The listing builds one solid part. Answer for the finished solid, in the listing's coordinates (mm). A direction names the side the tool comes from. Give positions to 0.01 mm unless a question says otherwise; leave off trailing zeros. Order: outer loops, then holes, each group sorted by start corner. A loop starts at its lowest first (then second) coordinate and runs counter-clockwise, first axis right, second up.
```python
from build123d import *

# Parameters (mm, degrees)
SM_BASE_FLANGE_1_DEPTH = 15
CUT_EXTRUDE_1_DEPTH    = 10
FILLET_1_R             = 5


# Sheet-metal steps are written as plain solids
with BuildPart() as part:
    # Sketch 1 → 基体-法兰1 (new, symmetric)
    with BuildSketch(Plane.XY):
        with BuildLine():
            Line((204, 72), (204, 6))
            ThreePointArc((204, 6), (202.242640687, 1.757359313), (198, 0))
            Line((198, 0), (-198, 0))
            ThreePointArc((-198, 0), (-202.242640687, 1.757359313), (-204, 6))
            Line((-204, 6), (-204, 72))
            Line((-204, 72), (-210, 72))
            Line((-210, 72), (-210, 6))
            ThreePointArc((-210, 6), (-206.485281374, -2.485281374), (-198, -6))
            Line((-198, -6), (198, -6))
            ThreePointArc((198, -6), (206.485281374, -2.485281374), (210, 6))
            Line((210, 6), (210, 72))
            Line((210, 72), (204, 72))
        make_face()
    extrude(amount=SM_BASE_FLANGE_1_DEPTH, both=True)

    # 草图6 → 切除-拉伸1 (cut)
    with BuildSketch(Plane.XZ.offset(6)):
        with BuildLine():
            Line((13.5, 7.5), (124.5, 7.5))
            ThreePointArc((124.5, 7.5), (132, 0), (124.5, -7.5))
            Line((124.5, -7.5), (13.5, -7.5))
            ThreePointArc((13.5, -7.5), (6, 0), (13.5, 7.5))
        make_face()
        with BuildLine():
            Line((-13.5, 7.5), (-124.5, 7.5))
            ThreePointArc((-124.5, 7.5), (-132, 0), (-124.5, -7.5))
            Line((-124.5, -7.5), (-13.5, -7.5))
            ThreePointArc((-13.5, -7.5), (-6, 0), (-13.5, 7.5))
        make_face()
    extrude(amount=-CUT_EXTRUDE_1_DEPTH, mode=Mode.SUBTRACT)

    # 圆角1
    fillet_1_edges = [part.edges().sort_by_distance(p)[0] for p in [
        (-207, 72, -15),
        (207, 72, -15),
        (-207, 72, 15),
        (207, 72, 15),
    ]]
    fillet(fillet_1_edges, radius=FILLET_1_R)


solid = part.part
```
1) Straight lines are drawn through the part: probe 1 along X at (y, z) = (17.5, -12); probe 2 along Z at (x, y) = (68, -1); probe 3 along X at (y, z) = (5, -3.25). For each, find the intervals that lie inside material, in ascending order.
Geometry says:
probe 1: x = -210 to -204, 204 to 210
probe 2: z = -15 to -7.5, 7.5 to 15
probe 3: x = -209.96 to -203.92, 203.92 to 209.96
2) Find section D-D (x = 161). Write down the section's boundary in (y, z).
Geometry says:
outline: (-6, -15) - (0, -15) - (0, 15) - (-6, 15) - close
3) Find section B-B (z = 0). Write down the section's boundary in (x, y), then the cut area to 3 significant figures.
Geometry says:
outline: (-210, 6) arc R12 ccw to (-198, -6) - (-132, -6) - (-132, 0) - (-198, 0) arc R6 cw to (-204, 6) - (-204, 72) - (-210, 72) - close; (-6, -6) - (6, -6) - (6, 0) - (-6, 0) - close; (132, -6) - (198, -6) arc R12 ccw to (210, 6) - (210, 72) - (204, 72) - (204, 6) arc R6 cw to (198, 0) - (132, 0) - close
area: 1,830 mm2
4) A tool of negligible diameter and unlimited length cuts with its end or side. For faces 1 (the cylindrical face through (-206.58, -2.39, 0.21)), 2 (the cylindrical face through (-132, -3, 0)), 3 (the flat face through (204, 39, 0)), from which of +Z, -Z, +X, -X, +Y, -Y can it reach the whole face along a straight path? Write none if from no direction.
Geometry says:
face 1: +Z, -Z, -X, -Y
face 2: +Y, -Y
face 3: +Z, -Z, +Y
5) Find section A-A (y = 59.5). Write down the section's boundary in (x, z), then the cut area to 3 significant figures.
Geometry says:
outline: (-210, -15) - (-204, -15) - (-204, 15) - (-210, 15) - close; (204, -15) - (210, -15) - (210, 15) - (204, 15) - close
area: 360 mm2
6) For a pull along Z with two mould halves and no side action, classify faces 4 (the cylindrical face through (132, -3, 0)), 5 (the cylindrical face through (-6, -3, 0)), 6 (the flat face through (210, 39, 0)), 7 (the flat face through (-1, -2, -15)) as +Z half, -Z half, draft (parallel to the pull), parting line (faces both ways), or undercut.
Geometry says:
face 4: undercut
face 5: undercut
face 6: draft
face 7: -Z half
7) Find section C-C (x = 86.5). Write down the section's boundary in (y, z), then the cut area to 3 significant figures.
Geometry says:
outline: (-6, -15) - (0, -15) - (0, -7.5) - (-6, -7.5) - close; (-6, 7.5) - (0, 7.5) - (0, 15) - (-6, 15) - close
area: 90.0 mm2
8) Given P1, Ø15, axis at x = -11, z = 3.5, coming from the +Y side, flat-ended and moving along its own axis, determine where the tip first touches the part or whether it passes through.
Geometry says:
P1: stops at y = 0
